Autodesk Inventor part; units mm, degrees
ref_plane "YZ Plane" through (0, 0, 0) normal (1, 0, 0) x (0, 1, 0)
ref_plane "XZ Plane" through (0, 0, 0) normal (0, 1, 0) x (-1, 0, 0)
ref_plane "XY Plane" through (0, 0, 0) normal (0, 0, 1) x (1, 0, 0)
sketch "Sketch1" plane through (0, 0, 0) normal (0, 1, 0) x (-1, 0, 0)
  line L0 (-15.25, 13.2) -> (15.25, 13.2)
  line L1 (15.25, 13.2) -> (15.25, -13.2)
  line L2 (15.25, -13.2) -> (-15.25, -13.2)
  line L3 (-15.25, -13.2) -> (-15.25, 13.2)
  line L4 (-15.25, 13.2) -> (15.25, -13.2) construction
  line L5 (15.25, 13.2) -> (-15.25, -13.2) construction
  point P0 (0, 0)
  dimension "d0" = 30.5
  dimension "d1" = 26.4
extrude "Extrusion1" add sketch "Sketch1" along normal blind 16.2
sketch "Sketch2" plane through (0, 16.2, 0) normal (0, 1, 0) x (1, 0, 0)
  circle A0 centre (3.75, 1.7) radius 8.5
  line L0 (15.25, -13.2) -> (15.25, 13.2)
  line L1 (15.25, 13.2) -> (-15.25, 13.2)
  point P0 (0, 0)
  dimension "d4" = 17
  dimension "d5" = 11.5
  dimension "d6" = 11.5
extrude "Extrusion2" add sketch "Sketch2" along normal blind 3.5
sketch "Sketch3" plane through (0, 0, 0) normal (0, -1, 0) x (1, 0, 0)
  line L0 (-15.25, 13.2) -> (-15.25, -13.2)
  line L1 (-15.25, 13.2) -> (-5.65, 13.2)
  line L2 (-5.65, 13.2) -> (-5.65, 3.6)
  line L3 (-5.65, 3.6) -> (-15.25, 3.6)
  line L4 (-15.25, 3.6) -> (-15.25, 13.2)
  point P0 (0, 0)
  dimension "d9" = 9.6
  dimension "d10" = 9.6
extrude "Extrusion3" cut sketch "Sketch3" against normal blind 5.5
sketch "Sketch4" plane through (0, 5.5, 0) normal (0, -1, 0) x (1, 0, 0)
  line L0 (-15.25, 13.2) -> (-5.65, 13.2)
  line L1 (-15.25, 3.6) -> (-15.25, 13.2)
  line L2 (-5.65, 3.6) -> (-15.25, 3.6)
  line L3 (-5.65, 13.2) -> (-5.65, 3.6)
  circle A0 centre (-10.45, 8.4) radius 4.8
  point P0 (0, 0)
  dimension "d13" = 9.6
extrude "Extrusion4" add sketch "Sketch4" along normal blind 9.6 contours A0
sketch "Sketch5" plane through (0, 0, 0) normal (0, -1, 0) x (1, 0, 0)
  line L0 (-15.25, -13.2) -> (15.25, -13.2)
  line L1 (15.25, -13.2) -> (15.25, 13.2)
  line L2 (-2.25, -7.7) -> (10.75, -7.7)
  line L3 (10.75, -7.7) -> (10.75, 4.3)
  line L4 (10.75, 4.3) -> (-2.25, 4.3)
  line L5 (-2.25, 4.3) -> (-2.25, -7.7)
  arc A0 (12.75, 0.5759) -> (12.75, 4.0241) centre (13.05, 2.3) ccw
  arc A1 (2.0729, -9.7) -> (5.4271, -9.7) centre (3.75, -10.2) ccw
  arc A2 (5.2508, 6.3) -> (2.2492, 6.3) centre (3.75, 7.2) ccw
  arc A3 (-4.25, -2.7639) -> (-4.25, -5.6361) centre (-5.25, -4.2) ccw
  line L6 (12.75, -9.7) -> (5.4271, -9.7)
  line L7 (2.0729, -9.7) -> (-4.25, -9.7)
  line L8 (-15.25, 3.6) -> (-15.25, -13.2)
  line L9 (15.25, 13.2) -> (-5.65, 13.2)
  line L10 (-4.25, 6.3) -> (2.2492, 6.3)
  line L11 (5.2508, 6.3) -> (12.75, 6.3)
  line L12 (12.75, 6.3) -> (12.75, 4.0241)
  line L13 (12.75, 0.5759) -> (12.75, -9.7)
  line L14 (-4.25, -9.7) -> (-4.25, -5.6361)
  line L15 (-4.25, -2.7639) -> (-4.25, 6.3)
  point P0 (0, 0)
  dimension "d16" = 17
  dimension "d17" = 16
  dimension "d23" = 3.5
  dimension "d24" = 3.5
  dimension "d25" = 3.5
  dimension "d26" = 3.5
  dimension "d27" = 11.5
  dimension "d28" = 3
  dimension "d29" = 9
  dimension "d30" = 10
  dimension "d31" = 11.5
  dimension "d32" = 6
  dimension "d33" = 2.2
  dimension "d34" = 15.5
extrude "Extrusion5" add sketch "Sketch5" along normal blind 6
sketch "Sketch6" plane through (0, -6, 0) normal (0, -1, 0) x (1, 0, 0)
  line L0 (-2.25, -7.7) -> (-2.25, 4.3)
  line L1 (-2.25, 4.3) -> (10.75, 4.3)
  line L2 (10.75, 4.3) -> (10.75, -7.7)
  line L3 (10.75, -7.7) -> (-2.25, -7.7)
  line L4 (5.4271, -9.7) -> (12.75, -9.7)
  line L5 (12.75, -9.7) -> (12.75, 0.5759)
  arc A0 (12.75, 0.5759) -> (12.75, 4.0241) centre (13.05, 2.3) ccw
  line L6 (12.75, 4.0241) -> (12.75, 6.3)
  line L7 (12.75, 6.3) -> (5.2508, 6.3)
  arc A1 (5.2508, 6.3) -> (2.2492, 6.3) centre (3.75, 7.2) ccw
  line L8 (2.2492, 6.3) -> (-4.25, 6.3)
  line L9 (-4.25, 6.3) -> (-4.25, -2.7639)
  arc A2 (-4.25, -2.7639) -> (-4.25, -5.6361) centre (-5.25, -4.2) ccw
  line L10 (-4.25, -5.6361) -> (-4.25, -9.7)
  line L11 (-4.25, -9.7) -> (2.0729, -9.7)
  arc A3 (2.0729, -9.7) -> (5.4271, -9.7) centre (3.75, -10.2) ccw
  circle A4 centre (3.75, 7.2) radius 0.9
  circle A5 centre (13.05, 2.3) radius 0.9
  circle A6 centre (3.75, -10.2) radius 0.9
  circle A7 centre (-5.25, -4.2) radius 0.9
  point P0 (0, 0)
  dimension "d35" = 1.8
  dimension "d36" = 1.8
  dimension "d37" = 1.8
extrude "Extrusion6" cut sketch "Sketch6" against normal blind 6 contours A4 | A5 | A6 | A7
sketch "Sketch7" plane through (0, 0, 0) normal (0, -1, 0) x (1, 0, 0)
  circle A0 centre (-5.25, -8.7) radius 0.65
  circle A1 centre (12.25, -1.2) radius 0.65
  line L0 (-15.25, -13.2) -> (15.25, -13.2)
  line L1 (15.25, -13.2) -> (15.25, 13.2)
  point P0 (0, 0)
  dimension "d40" = 1.3
  dimension "d41" = 1.3
  dimension "d42" = 12
  dimension "d43" = 3
  dimension "d44" = 4.5
  dimension "d45" = 20.5
extrude "Extrusion7" add sketch "Sketch7" along normal blind 8.7
ref_plane "Arbeitsebene1" through (0, 0, -13.2) normal (-1, 0, 0) x (0, 0, 1)
properties part number "102_Z_Focus_CCTV_Camera"
Geometry: final body of the model. Coordinates: model frame, mm. A direction names the side the tool comes from. Round coordinates to 2 decimals unless told otherwise and drop trailing zeros. Loops run counter-clockwise (first coordinate to the right, second up) from the corner with the lowest first, then second, coordinate; pieces in that order, holes last. Notation, with made-up numbers: (37, 9.25) - (46, 9.25) arc R22 ccw to (46, 39.25) - close; hole circle Ø1 at (44.5, 19). An arc over 180 degrees is marked (long way). Write each question's results on one line, items separated by ' | '. Start each with the question number.
1) Cut plane B-B on x = 9.5. Return loops of the section in (y, z), then the cut area to 4 significant figures.
2) Mould query, pull axis Z, two halves, no side actions, for faces 5 (the face through (-6.15, -3.04, -4.16)), 6 (the face through (0, 8, 13.2)), 7 (the face through (-7, 5.5, 12)). Classes: released by +Z, released by -Z, zero draft, split by the parting line, or undercut.
3) Cut plane A-A on y = -2.5. Return loops of the section in (x, z), then the cut area to 3 significant figures.
4) Line query: probe 1 along Z at (x, y) = (3.75, -2.8); probe 2 along Z at (x, y) = (13.05, -2.35); probe 3 along X at (y, z) = (-2.25, -8). Output: solid intervals per line, ascending. Write a range as [from, to].
5) Cut plane C-C on z = 11. Return loops of the section in (x, y).
6) Access query for faces 1 (the face through (-2.515, 17.926, 4.045)), 2 (the face through (12.75, -3, -6)), 3 (the face through (-4.25, -3, -8)), 4 (the face through (-6.6, 5.5, 4.6)). Directions: +Z, -Z, +X, -X, +Y, -Y. A direction counts if a zero-diameter tool reaches every point of the face in a straight line with its end or side. Return the directions, or none.
7) Cut plane D-D on x = 1. Return loops of the section in (y, z).
8) First-contact query: P1, Ø1.4, axis at x = 4, z = -10.5, coming from the -Y side; P2, Ø1, axis at x = -5.5, z = 5.5, coming from the +Y side; P3, Ø2.5, axis at x = -12.5, y = 2, coming from the +Z side. Flat tips, straight axial feed; report the tip coordinate or a pass-through.
Verdict:
1) outline: (-6, -9.7) - (0, -9.7) - (0, -13.2) - (16.2, -13.2) - (16.2, -7.96) - (19.7, -7.96) - (19.7, 4.56) - (16.2, 4.56) - (16.2, 13.2) - (0, 13.2) - (0, 6.3) - (-6, 6.3) - (-6, 4.3) - (0, 4.3) - (0, -7.7) - (-6, -7.7) - close | area: 495.5 mm2
2) face 5: undercut | face 6: released by +Z | face 7: zero draft
3) outline: circle Ø9.6 at (-10.45, 8.4); circle Ø1.3 at (-5.25, -8.7); (-4.25, -9.7) - (2.07, -9.7) arc R1.75 ccw (long way) to (5.43, -9.7) - (12.75, -9.7) - (12.75, -1.62) arc R0.65 ccw to (12.75, -0.78) - (12.75, 0.58) arc R1.75 ccw (long way) to (12.75, 4.02) - (12.75, 6.3) - (5.25, 6.3) arc R1.75 ccw (long way) to (2.25, 6.3) - (-4.25, 6.3) - (-4.25, -2.76) arc R1.75 ccw (long way) to (-4.25, -5.64) - close; hole circle Ø1.8 at (-5.25, -4.2); hole (-2.25, -7.7) - (10.75, -7.7) - (10.75, 4.3) - (-2.25, 4.3) - close; hole circle Ø1.8 at (3.75, -10.2); hole circle Ø1.8 at (3.75, 7.2); hole circle Ø1.8 at (13.05, 2.3) | area: 208 mm2
4) probe 1: z = [-11.95, -11.1], [-9.3, -7.7], [4.3, 6.3], [8.1, 8.95] | probe 2: z = [0.55, 1.4], [3.2, 4.05] | probe 3: x = [-4.25, 12.75]
5) outline: (-15.25, 5.5) - (-14.48, 5.5) - (-14.48, -4.1) - (-6.42, -4.1) - (-6.42, 5.5) - (-5.65, 5.5) - (-5.65, 0) - (15.25, 0) - (15.25, 16.2) - (-15.25, 16.2) - close
6) face 1: +Y | face 2: -Z, +X, -Y | face 3: -Z, -Y | face 4: -Y
7) outline: (-6, -9.7) - (0, -9.7) - (0, -13.2) - (16.2, -13.2) - (16.2, -9.74) - (19.7, -9.74) - (19.7, 6.34) - (16.2, 6.34) - (16.2, 13.2) - (0, 13.2) - (0, 6.3) - (-6, 6.3) - (-6, 4.3) - (0, 4.3) - (0, -7.7) - (-6, -7.7) - close
8) P1: stops at y = -6 | P2: stops at y = 16.2 | P3: stops at z = 13.13
